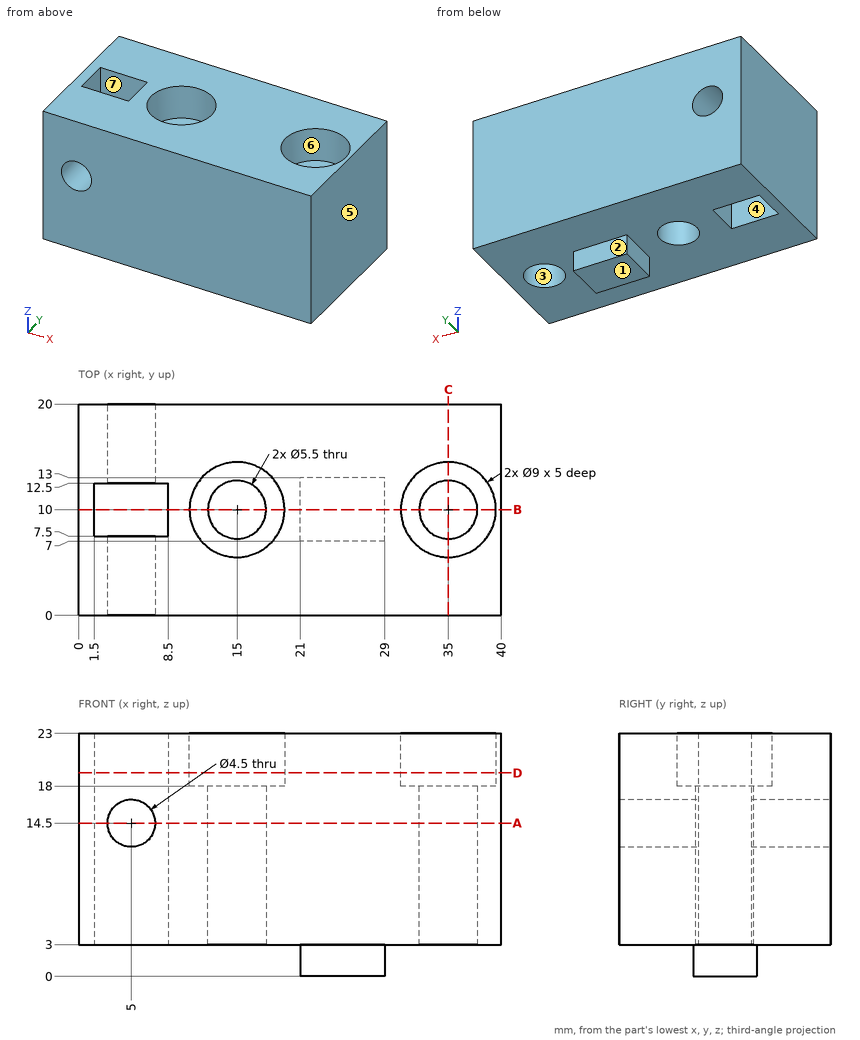
Part print with two shaded views. Sizes in mm from the minimum x, y, z corner. A direction names the side the tool comes from. Give positions to 0.01 mm unless a question says otherwise; leave off trailing zeros. Order: outer loops, then holes, each group sorted by start corner. A loop starts at its lowest first (then second) coordinate and runs counter-clockwise, first axis right, second up.
(1) Saw through at B-B, the plane y = 10. Give the cut face in (x, z), then the cut area to 3 significant figures.
(2) Saw through at A-A, the plane z = 14.5. Give the cut face in (x, y), then the cut area to 3 significant figures.
(3) Mould opens along Y. For the marked faces 1, 2, 3 and 4 say: released by +Y, released by -Y, zero draft, split by the parting line, or undercut.
(4) Flat gauge pins, fed straight in: pin 1 (11.5 mm diameter, centred on x = 35, y = 10, fed in from -Z); pin 2 (4.5 mm diameter, centred on x = 36.5, y = 11, fed in from +Z); pin 3 (1.5 mm diameter, centred on y = 11.5, z = 2, fed in from +X). Where does each tip first touch, or does it go through?
(5) Saw through at C-C, the plane x = 35. Give the cut face in (y, z), then the cut area to 4 significant figures.
(6) Drill centre lines: L1, parallel to Y at x = 15, z = 6.75; L2, parallel to X at y = 15, z = 14.5; L3, parallel to Z at x = 5, y = 5.5. Where is each one in solid material? Low to high.
(7) Saw through at D-D, the plane z = 19.25. Give the cut face in (x, y).
(8) Tool access for the marked faces 5, 6 and 7: list every direction of +Z, -Z, +X, -X, +Y, -Y with a clear straight run to the whole face (end or side of a thin tool).
Results found:
1. outline: (0, 3) - (1.5, 3) - (1.5, 23) - (0, 23) - close; (8.5, 3) - (12.25, 3) - (12.25, 18) - (10.5, 18) - (10.5, 23) - (8.5, 23) - close; (17.75, 3) - (21, 3) - (21, 0) - (29, 0) - (29, 3) - (32.25, 3) - (32.25, 18) - (30.5, 18) - (30.5, 23) - (19.5, 23) - (19.5, 18) - (17.75, 18) - close; (37.75, 3) - (40, 3) - (40, 23) - (39.5, 23) - (39.5, 18) - (37.75, 18) - close
1. area: 429 mm2
2. outline: (0, 0) - (2.75, 0) - (2.75, 7.5) - (1.5, 7.5) - (1.5, 12.5) - (2.75, 12.5) - (2.75, 20) - (0, 20) - close; (7.25, 0) - (40, 0) - (40, 20) - (7.25, 20) - (7.25, 12.5) - (8.5, 12.5) - (8.5, 7.5) - (7.25, 7.5) - close; hole circle Ø5.5 at (15, 10); hole circle Ø5.5 at (35, 10)
2. area: 650 mm2
3. face 1: zero draft
3. face 2: released by +Y
3. face 3: undercut
3. face 4: undercut
4. pin 1: stops at z = 3
4. pin 2: stops at z = 18
4. pin 3: stops at x = 29
5. outline: (0, 3) - (7.25, 3) - (7.25, 18) - (5.5, 18) - (5.5, 23) - (0, 23) - close; (12.75, 3) - (20, 3) - (20, 23) - (14.5, 23) - (14.5, 18) - (12.75, 18) - close
5. area: 272.5 mm2
6. L1: y = 0 to 7.25, 12.75 to 20
6. L2: x = 0 to 2.75, 7.25 to 40
6. L3: z = 3 to 12.25, 16.75 to 23
7. outline: (0, 0) - (40, 0) - (40, 20) - (0, 20) - close; hole (1.5, 7.5) - (8.5, 7.5) - (8.5, 12.5) - (1.5, 12.5) - close; hole circle Ø9 at (15, 10); hole circle Ø9 at (35, 10)
8. face 5: +Z, -Z, +X, +Y, -Y
8. face 6: +Z
8. face 7: +Z, -Z
